Design review of the part built by this model. Coordinates are the model's own, in mm. Coordinates: 2 decimals unless noted, no trailing zeros. Loops run counter-clockwise (first coordinate to the right, second up) from the corner with the lowest first, then second, coordinate; pieces in that order, holes last. Notation, with made-up numbers: (27, 59.25) -> (52, 59.25) arc R25 cw to (52, 89.25) -> close; hole circle Ø10 at (35.5, 50). An arc over 180 degrees is marked (long way). Use a Markdown table: item, result. Add a question column.
Q1. Clearance check with flat-ended pins moving along their axes: pin 1 Ø1.5 at (x, y) = (28.5, 2) entering from -Z; pin 2 Ø0.9 at (y, z) = (2, 29.5) entering from -X; pin 3 Ø5 at (x, z) = (-21.21, -21.21) entering from +Y; pin 4 Ø12 at (x, z) = (-5, 19) entering from +Y. State where each tip first meets the part, or that it passes through.
Q2. For probe 1 along Z at (x, y) = (27, 1.95); probe 2 along Z at (x, y) = (5, 0.95); probe 3 along X at (y, z) = (1, -23), list the stretches that pass through material, from the lowest coordinate up.
Q3. Take a section at B-B on x = 5. Write out the cut boundary in (y, z).
Q4. Take a section at C-C on y = 0.6. Count the separate pieces of the cut face and the enclosed holes in it, plus the area to 3 significant figures.
Q5. Take a section at D-D on x = 24. Write out the cut boundary in (y, z).
Q6. Take a section at A-A on z = -1. Write out the cut boundary in (x, y).
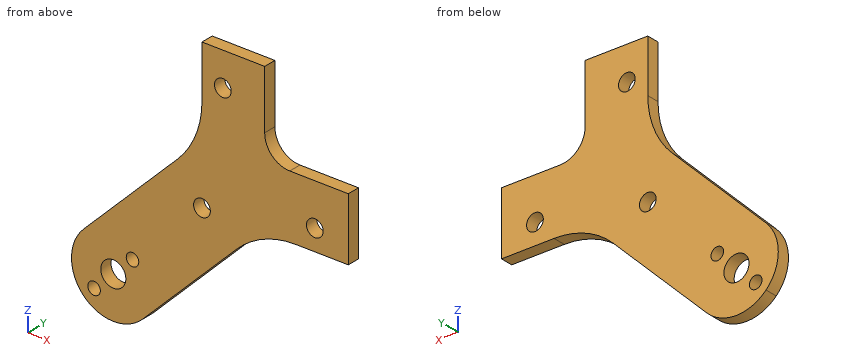
Autodesk Inventor part; units mm, degrees
ref_plane "YZ Plane" through (0, 0, 0) normal (1, 0, 0) x (0, 1, 0)
ref_plane "XZ Plane" through (0, 0, 0) normal (0, 1, 0) x (-1, 0, 0)
ref_plane "XY Plane" through (0, 0, 0) normal (0, 0, 1) x (1, 0, 0)
sketch "Sketch23" plane through (0, 0, 0) normal (0, 1, 0) x (-1, 0, 0)
  line L0 (0, -7) -> (0, 42)
  line L1 (7, 0) -> (-42, 0)
  line L2 (0, 0) -> (-35, 0)
  line L3 (-35, 0) -> (-35, 35)
  line L4 (-35, 35) -> (0, 35)
  line L5 (0, 35) -> (0, 0)
  line L6 (0, 0) -> (-35, 35) construction
  point P0 (0, 0)
  dimension "d213" = 35
  dimension "d214" = 35
extrude "Extrusion14" add sketch "Sketch23" along normal blind 3
sketch "Sketch24" plane through (0, 3, 0) normal (0, 1, 0) x (1, 0, 0)
  line L0 (35, 0) -> (0, 0)
  line L1 (0, 0) -> (0, -35)
  line L2 (0, -35) -> (35, -35)
  line L3 (35, -35) -> (35, 0)
  line L4 (-41.7276, 41.7276) -> (35, -35) construction
  line L5 (-35.3553, 21.2132) -> (-21.2132, 35.3553)
  line L6 (-21.2132, 35.3553) -> (14.1421, 0)
  line L7 (35, 0) -> (0, 0)
  line L8 (0, -14.1421) -> (-35.3553, 21.2132)
  line L9 (-23.915, -23.915) -> (42.6519, 42.6519) construction
  dimension "d217" = 45
  dimension "d218" = 20
  dimension "d219" = 40
extrude "Extrusion15" add sketch "Sketch24" against normal blind 3 contours L0 L1 L8 L5 L6
sketch "Sketch36" plane through (0, 3, 0) normal (0, 1, 0) x (1, 0, 0)
  line L0 (-35.3553, 21.2132) -> (0, -14.1421)
  line L1 (14.1421, 0) -> (-21.2132, 35.3553)
  line L2 (-21.2132, 35.3553) -> (-35.3553, 21.2132)
  line L3 (-24.0416, 32.5269) -> (-32.5269, 24.0416)
  line L4 (20, -20) -> (32, -20)
  line L5 (-18.4468, 18.4468) -> (20, -20) construction
  line L6 (-49.4264, 0) -> (49.0711, 0)
  line L7 (0, 49.4264) -> (0, -49.0711)
  line L8 (35, 0) -> (14.1421, 0)
  line L9 (0, -14.1421) -> (0, -35)
  line L10 (35, -35) -> (35, 0)
  line L11 (0, -35) -> (35, -35)
  point P0 (0, 0)
  point P1 (-18.3848, 9.8995)
  point P2 (0, -32)
  point P3 (32, 0)
  point P4 (-9.8995, 18.3848)
  point P5 (-21.2132, 21.2132)
  dimension "d311" = 45
  dimension "d312" = 10
hole "Hole17" at (-21.2132, 3, -21.2132) direction (0, -1, 0) diameter 6 end through all
sketch "Sketch37" plane through (0, 3, 0) normal (0, 1, 0) x (1, 0, 0)
  circle A0 centre (-21.2132, 21.2132) radius 3
  line L0 (14.1421, 0) -> (-21.2132, 35.3553)
  line L1 (-21.2132, 35.3553) -> (-35.3553, 21.2132)
  line L2 (-35.3553, 21.2132) -> (0, -14.1421)
  line L3 (-34.5369, 34.5369) -> (-7.0609, 7.0609) construction
  line L4 (-38.7653, 3.6611) -> (1.6595, 44.0859) construction
  line L5 (-53.5184, 0) -> (49.7531, 0)
  line L6 (0, 59.903) -> (0, -50.8172)
  line L7 (35, 0) -> (14.1421, 0)
  line L8 (0, -14.1421) -> (0, -35)
  line L9 (35, -35) -> (35, 0)
  line L10 (0, -35) -> (35, -35)
  point P0 (0, 0)
  point P1 (32, 0)
  point P2 (0, -32)
  point P3 (-25.8094, 25.8094)
  point P4 (-16.617, 16.617)
  dimension "d321" = 45
  dimension "d322" = 45
  dimension "d323" = 6.5
  dimension "d324" = 6.5
hole "Hole18" at (-25.8094, 3, -25.8094) at (-16.617, 3, -16.617) direction (0, -1, 0) diameter 3 end through all
fillet "Fillet15" radius 10 2 edges at (-35.3553, 1.5, -21.2132) (-21.2132, 1.5, -35.3553)
fillet "Fillet18" radius 20 2 edges at (14.1421, 1.5, 0) (0, 1.5, 14.1421)
sketch "Sketch39" plane through (0, 3, 0) normal (0, 1, 0) x (1, 0, 0)
  circle A0 centre (-21.2132, 21.2132) radius 3
  circle A1 centre (-16.617, 16.617) radius 1.5
  circle A2 centre (-25.8094, 25.8094) radius 1.5
  arc A3 (-14.1421, 28.2843) -> (-28.2843, 14.1421) centre (-21.2132, 21.2132) ccw
  line L0 (-28.2843, 14.1421) -> (-5.8579, -8.2843)
  arc A4 (0, -22.4264) -> (-5.8579, -8.2843) centre (-20, -22.4264) ccw
  line L1 (0, -22.4264) -> (0, -35)
  line L2 (35, 0) -> (22.4264, 0)
  arc A5 (8.2843, 5.8579) -> (22.4264, 0) centre (22.4264, 20) ccw
  line L3 (8.2843, 5.8579) -> (-14.1421, 28.2843)
  line L4 (26.8786, -26.8786) -> (-35.1686, 35.1686) construction
  line L5 (-58.6564, 0) -> (50.6094, 0)
  line L6 (0, 49.4264) -> (0, -49.0711)
  line L7 (-9.3628, 33.0636) -> (-43.047, -0.6206) construction
  line L8 (0, -35) -> (35, -35)
  line L9 (35, -35) -> (35, 0)
  point P0 (0, 0)
  point P1 (0, -32)
  point P2 (32, 0)
  point P3 (0, 0)
  dimension "d339" = 45
  dimension "d340" = 30
hole "Hole19" at (0, 3, 0) direction (0, -1, 0) diameter 4 end through all
sketch "Sketch40" plane through (0, 3, 0) normal (0, 1, 0) x (1, 0, 0)
  circle A0 centre (0, 0) radius 2
  circle A1 centre (-25.8094, 25.8094) radius 1.5
  circle A2 centre (-16.617, 16.617) radius 1.5
  circle A3 centre (-21.2132, 21.2132) radius 3
  arc A4 (-14.1421, 28.2843) -> (-28.2843, 14.1421) centre (-21.2132, 21.2132) ccw
  line L0 (-28.2843, 14.1421) -> (-5.8579, -8.2843)
  arc A5 (0, -22.4264) -> (-5.8579, -8.2843) centre (-20, -22.4264) ccw
  line L1 (0, -22.4264) -> (0, -35)
  line L2 (0, -35) -> (35, -35)
  line L3 (35, -35) -> (35, 0)
  line L4 (35, 0) -> (22.4264, 0)
  arc A6 (8.2843, 5.8579) -> (22.4264, 0) centre (22.4264, 20) ccw
  line L5 (8.2843, 5.8579) -> (-14.1421, 28.2843)
  line L6 (35, -35) -> (15, -35)
  line L7 (15, -35) -> (15, -15)
  line L8 (15, -15) -> (35, -15)
  line L9 (35, -15) -> (35, -35)
  line L10 (0, -35) -> (35, -35)
  line L11 (35, -35) -> (35, 0)
  point P0 (0, 0)
  dimension "d394" = 15
  dimension "d395" = 15
extrude "Extrusion19" cut sketch "Sketch40" against normal blind 10 contours L3 L2 L7 L8
fillet "Fillet19" radius 6 1 edges at (15, 1.5, 15)
sketch "Sketch44" plane through (0, 3, 0) normal (0, 1, 0) x (1, 0, 0)
  line L0 (15, -35) -> (15, -21)
  arc A0 (21, -15) -> (15, -21) centre (21, -21) ccw
  line L1 (21, -15) -> (35, -15)
  line L2 (35, 0) -> (22.4264, 0)
  arc A1 (8.2843, 5.8579) -> (22.4264, 0) centre (22.4264, 20) ccw
  line L3 (8.2843, 5.8579) -> (-14.1421, 28.2843)
  arc A2 (-14.1421, 28.2843) -> (-28.2843, 14.1421) centre (-21.2132, 21.2132) ccw
  line L4 (-28.2843, 14.1421) -> (-5.8579, -8.2843)
  arc A3 (0, -22.4264) -> (-5.8579, -8.2843) centre (-20, -22.4264) ccw
  line L5 (0, -22.4264) -> (0, -35)
  circle A4 centre (-21.2132, 21.2132) radius 3
  circle A5 centre (-16.617, 16.617) radius 1.5
  circle A6 centre (-25.8094, 25.8094) radius 1.5
  circle A7 centre (0, 0) radius 2
  line L6 (35, -15) -> (35, 0)
  line L7 (0, -35) -> (15, -35)
  point P0 (0, 0)
  point P1 (27, -5)
  point P2 (5, -27)
  dimension "d383" = 5
  dimension "d385" = 5
hole "Hole22" at (27, 3, 5) at (5, 3, 27) direction (0, -1, 0) diameter 4 end through all
properties part number "quarter_upper"
Answer list:
| question | item | result |
|---|---|---|
| 1 | pin 1 | z = 0 |
| 1 | pin 2 | x = 0 |
| 1 | pin 3 | through |
| 1 | pin 4 | y = 3 |
| 2 | probe 1 | 0 to 3, 7 to 15 |
| 2 | probe 2 | -9.14 to 25, 29 to 35 |
| 2 | probe 3 | -31.05 to -23.62, -18.8 to -8.86 |
| 3 | outline | (0, -9.14) -> (3, -9.14) -> (3, 25) -> (0, 25) -> close; (0, 29) -> (3, 29) -> (3, 35) -> (0, 35) -> close |
| 4 | separate pieces | 1 |
| 4 | enclosed holes | 6 |
| 4 | area | 1,630 mm² |
| 5 | outline | (0, 0) -> (3, 0) -> (3, 15) -> (0, 15) -> close |
| 6 | outline | (-15.14, 0) -> (-1.73, 0) -> (-1.73, 3) -> (-15.14, 3) -> close; (1.73, 0) -> (16.18, 0) -> (16.18, 3) -> (1.73, 3) -> close |
